Part model, mm, in its own coordinate system. Face numbers are marked on the shaded views. A direction names the side the tool comes from. Give positions to 0.01 mm unless a question says otherwise; leave off trailing zeros. Write each loop counter-clockwise with the first axis right and the second up, starting at its lowest first coordinate (ties: lowest second). Pieces come first, ordered by that corner, then holes. Notation, with made-up numbers: M 28.25,2 L 62.25,2 A28 ccw 62.25,38 Z; hole C 37,23.25 d8. An arc over 180 degrees is marked long. Use a Markdown table: item, result. Add a question column.
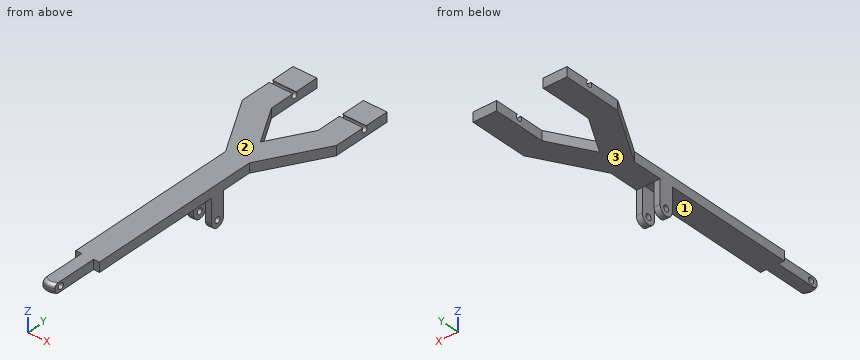
from build123d import *

# Parameters (mm, degrees)
BOSS_EXTRU_1_DEPTH      = 40
ENL_V_MAT_EXTRU_2_DEPTH = 972.24221049
ESQUISSE3_R             = 12.5
ENL_V_MAT_EXTRU_3_DEPTH = 50
CONG_1_R                = 15
ESQUISSE6_R             = 12.5
BOSS_EXTRU_2_DEPTH      = 50
ENL_V_MAT_EXTRU_4_DEPTH = 25
ESQUISSE7_R             = 12.5
ENL_V_MAT_EXTRU_5_DEPTH = 1038.379889384


with BuildPart() as part:
    # Esquisse1 → Boss.-Extru.1 (new body)
    with BuildSketch(Plane.XY):
        with BuildLine():
            Line((-50, -13.397459622), (-50, -900))
            ThreePointArc((-50, -900), (0, -950), (50, -900))
            Line((50, -900), (50, -13.397459622))
            Line((50, -13.397459622), (43.301270189, -25))
            ThreePointArc((43.301270189, -25), (0, -50), (-43.301270189, -25))
            Line((-43.301270189, -25), (-50, -13.397459622))
        make_face()
        with BuildLine():
            Line((-50, 0), (-50, -13.397459622))
            Line((-50, -13.397459622), (-43.301270189, -25))
            ThreePointArc((-43.301270189, -25), (0, -50), (43.301270189, -25))
            Line((43.301270189, -25), (50, -13.397459622))
            Line((50, -13.397459622), (50, 0))
            ThreePointArc((50, 0), (48.296291314, 12.940952255), (43.301270189, 25))
            ThreePointArc((43.301270189, 25), (0, 50), (-43.301270189, 25))
            ThreePointArc((-43.301270189, 25), (-48.296291314, 12.940952255), (-50, 0))
        make_face()
        with BuildLine():
            Line((-198.018765367, 242.978562467), (-50, -13.397459622))
            Line((-50, -13.397459622), (-50, 0))
            ThreePointArc((-50, 0), (-48.296291314, 12.940952255), (-43.301270189, 25))
            ThreePointArc((-43.301270189, 25), (0, 50), (43.301270189, 25))
            ThreePointArc((43.301270189, 25), (48.296291314, 12.940952255), (50, 0))
            Line((50, 0), (50, -13.397459622))
            Line((50, -13.397459622), (198.018765367, 242.978562467))
            Line((198.018765367, 242.978562467), (198.018765367, 492.978562467))
            Line((198.018765367, 492.978562467), (98.018765367, 492.978562467))
            Line((98.018765367, 492.978562467), (98.018765367, 392.978562467))
            Line((98.018765367, 392.978562467), (98.018765367, 342.978562467))
            Line((98.018765367, 342.978562467), (98.018765367, 269.773481711))
            Line((98.018765367, 269.773481711), (0, 100))
            Line((0, 100), (-98.018765367, 269.773481711))
            Line((-98.018765367, 269.773481711), (-98.018765367, 342.978562467))
            Line((-98.018765367, 342.978562467), (-98.018765367, 392.978562467))
            Line((-98.018765367, 392.978562467), (-98.018765367, 492.978562467))
            Line((-98.018765367, 492.978562467), (-198.018765367, 492.978562467))
            Line((-198.018765367, 492.978562467), (-198.018765367, 242.978562467))
        make_face()
    extrude(amount=BOSS_EXTRU_1_DEPTH)

    # Esquisse2 → Enlèv. mat.-Extru.2 (cut, through all)
    with BuildSketch(Plane(origin=(0, 0, 0), x_dir=(-1, 0, 0), z_dir=(0, 0, -1))):
        with BuildLine():
            ThreePointArc((50, -900), (43.301270189, -925), (25, -943.301270189))
            Line((25, -943.301270189), (25, -1037.943368981))
            Line((25, -1037.943368981), (50, -1037.943368981))
            Line((50, -1037.943368981), (50, -900))
        make_face()
        with BuildLine():
            ThreePointArc((-25, -943.301270189), (-43.301270189, -925), (-50, -900))
            Line((-50, -900), (-50, -1037.943368981))
            Line((-50, -1037.943368981), (-25, -1037.943368981))
            Line((-25, -1037.943368981), (-25, -943.301270189))
        make_face()
        with BuildLine():
            Line((-25, -752.632896004), (-50, -752.632896004))
            Line((-50, -752.632896004), (-50, -900))
            ThreePointArc((-50, -900), (-43.301270189, -925), (-25, -943.301270189))
            Line((-25, -943.301270189), (-25, -752.632896004))
        make_face()
        with BuildLine():
            Line((50, -752.632896004), (25, -752.632896004))
            Line((25, -752.632896004), (25, -943.301270189))
            ThreePointArc((25, -943.301270189), (43.301270189, -925), (50, -900))
            Line((50, -900), (50, -752.632896004))
        make_face()
    extrude(amount=-ENL_V_MAT_EXTRU_2_DEPTH, mode=Mode.SUBTRACT)

    # Esquisse3 → Enlèv. mat.-Extru.3 (cut)
    with BuildSketch(Plane(origin=(25, 0, 0), x_dir=(0, 0, -1), z_dir=(1, 0, 0))):
        with Locations((-20, -913.975598424)):
            Circle(ESQUISSE3_R)
    extrude(amount=-ENL_V_MAT_EXTRU_3_DEPTH, mode=Mode.SUBTRACT)

    # Congé1
    cong_1_edges = [part.edges().sort_by_distance(p)[0] for p in [
        (0, -950, 0),
        (0, -950, 40),
    ]]
    fillet(cong_1_edges, radius=CONG_1_R)

    # Esquisse6 → Boss.-Extru.2 (add, symmetric)
    with BuildSketch(Plane(origin=(0, 0, 0), x_dir=(0, 0, -1), z_dir=(1, 0, 0))):
        with BuildLine():
            Line((99.658431886, -139.909310173), (-10.672864852, -139.909310173))
            Line((-10.672864852, -139.909310173), (-10.672864852, -199.909310173))
            Line((-10.672864852, -199.909310173), (99.658431886, -199.909310173))
            ThreePointArc((99.658431886, -199.909310173), (129.658431886, -169.909310173), (99.658431886, -139.909310173))
        make_face()
        with Locations(Location((99.658431886, -169.909310173, 0), (0, 0, 180))):
            Circle(ESQUISSE6_R, mode=Mode.SUBTRACT)
    extrude(amount=BOSS_EXTRU_2_DEPTH, both=True)

    # Esquisse6 → Enlèv. mat.-Extru.4 (cut, symmetric)
    with BuildSketch(Plane(origin=(0, 0, 0), x_dir=(0, 0, -1), z_dir=(1, 0, 0))):
        with BuildLine():
            Line((99.658431886, -139.909310173), (-10.672864852, -139.909310173))
            Line((-10.672864852, -139.909310173), (-10.672864852, -199.909310173))
            Line((-10.672864852, -199.909310173), (99.658431886, -199.909310173))
            ThreePointArc((99.658431886, -199.909310173), (129.658431886, -169.909310173), (99.658431886, -139.909310173))
        make_face()
        with Locations(Location((99.658431886, -169.909310173, 0), (0, 0, 180))):
            Circle(ESQUISSE6_R, mode=Mode.SUBTRACT)
    extrude(amount=ENL_V_MAT_EXTRU_4_DEPTH, both=True, mode=Mode.SUBTRACT)

    # Esquisse7 → Enlèv. mat.-Extru.5 (cut, through all)
    with BuildSketch(Plane(origin=(198.018765367, 0, 0), x_dir=(0, 0, -1), z_dir=(1, 0, 0))):
        with Locations((-30, 382.978562467)):
            Circle(ESQUISSE7_R)
    extrude(amount=-ENL_V_MAT_EXTRU_5_DEPTH, mode=Mode.SUBTRACT)


solid = part.part
1. Flat gauge pins, fed straight in: pin 1 (1 mm diameter, centred on y = -150, z = 1, fed in from +X); pin 2 (12.5 mm diameter, centred on x = -31.5, z = -41, fed in from +Y); pin 3 (20 mm diameter, centred on x = -40.5, z = -62.5, fed in from -Y). Where does each tip first touch, or does it go through?
2. Cut at D-D (x = -71). Write the cut outline in (y, z).
3. Cut at A-A (z = -56). Write the cut outline in (x, y), then the cut area to 3 significant figures.
4. Cut at B-B (y = 203.5). Write the cut outline in (x, z).
5. Drill centre lines: probe 1 along X at (y, z) = (-156.5, -51.5); probe 2 along Y at (x, z) = (-39, -72.5); probe 3 along Y at (x, z) = (-157, 22.5). Where is each one in solid material? Low to high. Write a range as [from, to].
6. Cut at C-C (y = -808). Write the cut outline in (x, z), then the cut area to 3 significant figures.
7. Tool access for the marked faces 1, 2 and 3: list every direction of +Z, -Z, +X, -X, +Y, -Y with a clear straight run to the whole face (end or side of a thin tool).
A:
| question | item | result |
|---|---|---|
| 1 | pin 1 | stops at x = 50 |
| 1 | pin 2 | stops at y = -139.91 |
| 1 | pin 3 | stops at y = -199.91 |
| 2 | outline | M 22.98,0 L 222.98,0 L 222.98,40 L 22.98,40 Z |
| 3 | outline | M -50,-199.91 L -25,-199.91 L -25,-139.91 L -50,-139.91 Z; M 25,-199.91 L 50,-199.91 L 50,-139.91 L 25,-139.91 Z |
| 3 | area | 3,000 mm² |
| 4 | outline | M -175.23,0 L -59.76,0 L -59.76,40 L -175.23,40 Z; M 59.76,0 L 175.23,0 L 175.23,40 L 59.76,40 Z |
| 5 | probe 1 | x = [-50, -25], [25, 50] |
| 5 | probe 2 | y = [-199.91, -139.91] |
| 5 | probe 3 | y = [171.93, 372.98], [392.98, 492.98] |
| 6 | outline | M -25,0 L 25,0 L 25,40 L -25,40 Z |
| 6 | area | 2,000 mm² |
| 7 | face 1 | -Z, +X, -X, -Y |
| 7 | face 2 | +Z, +X, -X, +Y, -Y |
| 7 | face 3 | -Z, +X, -X, +Y |
